```python
from build123d import *

# Parameters (mm, degrees)
SKETCH2_W           = 98
SKETCH2_H           = 20
BOSS_EXTRUDE1_DEPTH = 42
SKETCH4_W           = 32
SKETCH4_H           = 4.7
CUT_EXTRUDE1_DEPTH  = 109.480412979
SKETCH6_R           = 4
CUT_EXTRUDE3_DEPTH  = 108.712998287
SKETCH7_R           = 15
CUT_EXTRUDE4_DEPTH  = 109.480412979


with BuildPart() as part:
    # Sketch2 → Boss-Extrude1 (new body)
    with BuildSketch(Plane.XY):
        with Locations((49, 10)):
            Rectangle(SKETCH2_W, SKETCH2_H)
    extrude(amount=BOSS_EXTRUDE1_DEPTH)

    # Sketch4 → Cut-Extrude1 (cut, through all)
    with BuildSketch(Plane(origin=(98, 0, 0), x_dir=(0, 0, -1), z_dir=(1, 0, 0))):
        with Locations((-21, 17.65)):
            Rectangle(SKETCH4_W, SKETCH4_H)
    extrude(amount=-CUT_EXTRUDE1_DEPTH, mode=Mode.SUBTRACT)

    # Sketch6 → Cut-Extrude3 (cut, through all)
    with BuildSketch(Plane(origin=(0, 15.3, 0), x_dir=(1, 0, 0), z_dir=(0, 1, 0))):
        with Locations(Location((11, -21, 0), (0, 0, 270))):
            Circle(SKETCH6_R)
        with Locations(Location((87, -21, 0), (0, 0, 90))):
            Circle(SKETCH6_R)
    extrude(amount=-CUT_EXTRUDE3_DEPTH, mode=Mode.SUBTRACT)

    # Sketch7 → Cut-Extrude4 (cut, through all)
    with BuildSketch(Plane.XY.offset(42)):
        with Locations((49, 0)):
            Circle(SKETCH7_R)
    extrude(amount=-CUT_EXTRUDE4_DEPTH, mode=Mode.SUBTRACT)


solid = part.part
```
Design review of the part built by this model. Coordinates are the model's own, in mm. A direction names the side the tool comes from. Coordinates: 2 decimals unless noted, no trailing zeros. Order: outer loops, then holes, each group sorted by start corner. A loop starts at its lowest first (then second) coordinate and runs counter-clockwise, first axis right, second up. Notation, with made-up numbers: (62, 6.5) - (78, 6.5) arc R26 ccw to (78, 32.5) - close; hole circle Ø11 at (23, 53). An arc over 180 degrees is marked (long way). One line per question, with ' | ' between items.
Q1. To check wall thickness, follow line 1 along Z through (x, y) = (87, 6.5); line 2 along X through (y, z) = (9.5, 21); line 3 along X through (y, z) = (5.75, 21). State the ranges of each line that lie inside material, in increasing order.
Answer key:
line 1: z = 0 to 17, 25 to 42 | line 2: x = 0 to 7, 15 to 37.39, 60.61 to 83, 91 to 98 | line 3: x = 0 to 7, 15 to 35.15, 62.85 to 83, 91 to 98
Q2. For faces 4 (the cylindrical face through (13.7, 7.76, 18.05)), 5 (the flat face through (50, 15.3, 21)), list the 3-axis set-ups (+Z, -Z, +X, -X, +Y, -Y) from which the entire face can be reached by the end or side of a thin tool; tool diameter is ignored.
Answer key:
face 4: +Y, -Y | face 5: +X, -X, +Y
Q3. Consider section B-B, the plane x = 87. Give the boundary of the cut face in (y, z), then the cut area to 3 significant figures.
Answer key:
outline: (0, 0) - (20, 0) - (20, 5) - (15.3, 5) - (15.3, 17) - (0, 17) - close; (0, 25) - (15.3, 25) - (15.3, 37) - (20, 37) - (20, 42) - (0, 42) - close | area: 567 mm2
Q4. Consider section C-C, the plane z = 18. Give the boundary of the cut face in (x, y), then the cut area to 3 significant figures.
Answer key:
outline: (0, 0) - (8.35, 0) - (8.35, 15.3) - (0, 15.3) - close; (13.65, 0) - (34, 0) arc R15 cw to (64, 0) - (84.35, 0) - (84.35, 15.3) - (13.65, 15.3) - close; (89.65, 0) - (98, 0) - (98, 15.3) - (89.65, 15.3) - close | area: 984 mm2
Q5. Consider section D-D, the plane x = 49. Give the boundary of the cut face in (y, z), then the cut area to 3 significant figures.
Answer key:
outline: (15, 0) - (20, 0) - (20, 5) - (15.3, 5) - (15.3, 37) - (20, 37) - (20, 42) - (15, 42) - close | area: 59.6 mm2
Q6. The part is to be moulded in two halves that separate along X. For faces 1 (the cylindrical face through (49, 15, 21)), 2 (the flat face through (48, 17, 0)), 3 (the flat face through (0, 8, 21)), say which applies: +X half, -X half, draft (parallel to the pull), parting line (faces both ways), or undercut.
Answer key:
face 1: undercut | face 2: draft | face 3: -X half
Q7. Clearance check with flat-ended pins moving along their axes: pin 1 Ø9 at (x, z) = (87, 21) entering from +Y; pin 2 Ø5 at (x, y) = (67, 17.5) entering from -Z; pin 3 Ø6 at (x, z) = (47, 26) entering from -Y. State where each tip first meets the part, or that it passes through.
Answer key:
pin 1: stops at y = 15.3 | pin 2: stops at z = 0 | pin 3: stops at y = 14.14
Q8. Consider section A-A, the plane y = 6.5. Give the boundary of the cut face in (x, z).
Answer key:
outline: (0, 0) - (35.48, 0) - (35.48, 42) - (0, 42) - close; (62.52, 0) - (98, 0) - (98, 42) - (62.52, 42) - close; hole circle Ø8 at (11, 21); hole circle Ø8 at (87, 21)
